```python
from build123d import *

# Parameters (mm, degrees)
SKETCH_1_W          = 100
SKETCH_1_H          = 100
EXTRUDE_1_DEPTH     = 1
SKETCH_2_R          = 1.75
CUT_EXTRUDE_1_DEPTH = 4
SKETCH_3_R          = 29
CUT_EXTRUDE_2_DEPTH = 4


with BuildPart() as part:
    # 草图1 → 凸台-拉伸1 (new body)
    with BuildSketch(Plane.XY):
        Rectangle(SKETCH_1_W, SKETCH_1_H)
    extrude(amount=EXTRUDE_1_DEPTH)

    # 草图2 → 切除-拉伸1 (cut)
    with BuildSketch(Plane.XY.offset(1)):
        with Locations((-42.5, 0)):
            Circle(SKETCH_2_R)
        with Locations((-30.0520382, 30.0520382)):
            Circle(SKETCH_2_R)
        with Locations((0, 42.5)):
            Circle(SKETCH_2_R)
        with Locations((30.0520382, 30.0520382)):
            Circle(SKETCH_2_R)
        with Locations((42.5, 0)):
            Circle(SKETCH_2_R)
        with Locations((30.0520382, -30.0520382)):
            Circle(SKETCH_2_R)
        with Locations((0, -42.5)):
            Circle(SKETCH_2_R)
        with Locations((-30.0520382, -30.0520382)):
            Circle(SKETCH_2_R)
    extrude(amount=-CUT_EXTRUDE_1_DEPTH, mode=Mode.SUBTRACT)

    # 草图3 → 切除-拉伸2 (cut)
    with BuildSketch(Plane.XY.offset(1)):
        Circle(SKETCH_3_R)
    extrude(amount=-CUT_EXTRUDE_2_DEPTH, mode=Mode.SUBTRACT)


solid = part.part
```
Here's how the part is built. I have some questions about the finished solid (model axes, mm). Coordinates: 2 decimals unless noted, no trailing zeros. Loops run counter-clockwise (first coordinate to the right, second up) from the corner with the lowest first, then second, coordinate; pieces in that order, holes last. Notation, with made-up numbers: (-7, -35) -> (50, -35) arc R27 cw to (50, -3) -> close; hole circle Ø3 at (17.5, 44). An arc over 180 degrees is marked (long way). Return JSON: item names as keys, results as strings.
1) Thinking about a two-plate mould opening in X: for faces 1 (the face through (13.38, -25.73, 0.51)), 2 (the face through (-31.44, -31.12, 0.51)), 3 (the face through (-23, 23, 1)), which applies, +X half, -X half, draft (parallel to the pull), parting line (faces both ways), or undercut?
Results below:
{"face 1": "undercut", "face 2": "undercut", "face 3": "draft"}
2) Will this pin go through, and if not, where does the flat tip stop? pin 1 (3 mm diameter, centred on x = 30.05, y = -30.05, fed in from +Z).
Results below:
{"pin 1": "through"}
3) If we section it at A-A, the plane x = 0: Write out the boundary of the cut face in (y, z).
Results below:
{"outline": "(-50, 0) -> (-44.25, 0) -> (-44.25, 1) -> (-50, 1) -> close; (-40.75, 0) -> (-29, 0) -> (-29, 1) -> (-40.75, 1) -> close; (29, 0) -> (40.75, 0) -> (40.75, 1) -> (29, 1) -> close; (44.25, 0) -> (50, 0) -> (50, 1) -> (44.25, 1) -> close"}
4) If we section it at B-B, the plane y = 42.5: Write out the boundary of the cut face in (x, z).
Results below:
{"outline": "(-50, 0) -> (-1.75, 0) -> (-1.75, 1) -> (-50, 1) -> close; (1.75, 0) -> (50, 0) -> (50, 1) -> (1.75, 1) -> close"}
5) I need wall thicknesses on line 1 (Y direction, x = 0, z = 0.9); line 2 (Y direction, x = 30, z = 0.5); line 3 (Y direction, x = 29.5, z = 0.45). Which ranges of each line are inside material? Lowest first, please. Write a range as from..to.
Results below:
{"line 1": "-50..-44.25, -40.75..-29, 29..40.75, 44.25..50", "line 2": "-50..-31.8, -28.3..28.3, 31.8..50", "line 3": "-50..-31.71, -28.39..28.39, 31.71..50"}
